Source: CAD feature listing. Evaluate the final solid. Frame: model axes, mm. Coordinates: 2 decimals unless noted, no trailing zeros. Loops run counter-clockwise (first coordinate to the right, second up) from the corner with the lowest first, then second, coordinate; pieces in that order, holes last. Notation, with made-up numbers: (-30, 16) -> (18, 16) arc R15 ccw to (18, 40) -> close; hole circle Ø1 at (85.25, 2.5). An arc over 180 degrees is marked (long way). Answer as CSV lines item,"result".
from build123d import *

# Parameters (mm, degrees)
SKETCH1_R                                    = 32
SKETCH1_R_2                                  = 8.25
BOSS_EXTRUDE1_DEPTH                          = 2
CSK_FOR_M3_HEX_SOCKET_COUNTERSUNK_HE_2_COUNT = 2
CSK_FOR_M3_HEX_SOCKET_COUNTERSUNK_HE_2_PITCH = 15
CSK_FOR_M3_HEX_SOCKET_COUNTERSUNK_HE_3_COUNT = 2
CSK_FOR_M3_HEX_SOCKET_COUNTERSUNK_HE_3_PITCH = 25.980762114
CSK_FOR_M3_HEX_SOCKET_COUNTERSUNK_HE_4_COUNT = 2
CSK_FOR_M3_HEX_SOCKET_COUNTERSUNK_HE_4_PITCH = 30
CSK_FOR_M3_HEX_SOCKET_COUNTERSUNK_HE_5_COUNT = 2
CSK_FOR_M3_HEX_SOCKET_COUNTERSUNK_HE_5_PITCH = 25.980762114
CSK_FOR_M3_HEX_SOCKET_COUNTERSUNK_HE_6_COUNT = 2
CSK_FOR_M3_HEX_SOCKET_COUNTERSUNK_HE_6_PITCH = 15
M3_CLEARANCE_HOLE1_D                         = 3.6


with BuildPart() as part:
    # Sketch1 → Boss-Extrude1 (new body)
    with BuildSketch(Plane(origin=(0, 0, 0), x_dir=(1, 0, 0), z_dir=(0, 1, 0))):
        with Locations(Location((0, 0, 0), (0, 0, 270))):
            Circle(SKETCH1_R)
        with Locations(Location((0, 0, 0), (0, 0, 270))):
            Circle(SKETCH1_R_2, mode=Mode.SUBTRACT)
    extrude(amount=BOSS_EXTRUDE1_DEPTH)

    # Sketch4 → CSK for M3 Hex Socket Countersunk Head Screw1 (revolve, cut)
    with BuildSketch(Plane(origin=(-7.5, 0, -12.990381057), x_dir=(0, 0, -1), z_dir=(1, 0, 0))):
        Polygon((0, 0), (0, 2), (1.7, 2), (1.7, 1.05), (2.75, 0), align=None)
    csk_for_m3_hex_socket_countersunk_head_s = revolve(axis=Axis((-7.5, -6.35, -12.990381057), (0, 1, 0)), mode=Mode.SUBTRACT)

    # CSK for M3 Hex Socket Countersunk He 2: CSK for M3 Hex Socket Countersunk Head Screw1 ×2
    with Locations(*[(i * CSK_FOR_M3_HEX_SOCKET_COUNTERSUNK_HE_2_PITCH, 0, 0) for i in range(1, CSK_FOR_M3_HEX_SOCKET_COUNTERSUNK_HE_2_COUNT)]):
        add(csk_for_m3_hex_socket_countersunk_head_s, mode=Mode.SUBTRACT)

    # CSK for M3 Hex Socket Countersunk He 3: CSK for M3 Hex Socket Countersunk Head Screw1 ×2
    with Locations(*[Vector(0.8660254037844752, 0, 0.49999999999993666) * (i * CSK_FOR_M3_HEX_SOCKET_COUNTERSUNK_HE_3_PITCH) for i in range(1, CSK_FOR_M3_HEX_SOCKET_COUNTERSUNK_HE_3_COUNT)]):
        add(csk_for_m3_hex_socket_countersunk_head_s, mode=Mode.SUBTRACT)

    # CSK for M3 Hex Socket Countersunk He 4: CSK for M3 Hex Socket Countersunk Head Screw1 ×2
    with Locations(*[Vector(0.5000000000000633, 0, 0.8660254037844022) * (i * CSK_FOR_M3_HEX_SOCKET_COUNTERSUNK_HE_4_PITCH) for i in range(1, CSK_FOR_M3_HEX_SOCKET_COUNTERSUNK_HE_4_COUNT)]):
        add(csk_for_m3_hex_socket_countersunk_head_s, mode=Mode.SUBTRACT)

    # CSK for M3 Hex Socket Countersunk He 5: CSK for M3 Hex Socket Countersunk Head Screw1 ×2
    with Locations(*[(0, 0, i * CSK_FOR_M3_HEX_SOCKET_COUNTERSUNK_HE_5_PITCH) for i in range(1, CSK_FOR_M3_HEX_SOCKET_COUNTERSUNK_HE_5_COUNT)]):
        add(csk_for_m3_hex_socket_countersunk_head_s, mode=Mode.SUBTRACT)

    # CSK for M3 Hex Socket Countersunk He 6: CSK for M3 Hex Socket Countersunk Head Screw1 ×2
    with Locations(*[Vector(-0.499999999999937, 0, 0.8660254037844751) * (i * CSK_FOR_M3_HEX_SOCKET_COUNTERSUNK_HE_6_PITCH) for i in range(1, CSK_FOR_M3_HEX_SOCKET_COUNTERSUNK_HE_6_COUNT)]):
        add(csk_for_m3_hex_socket_countersunk_head_s, mode=Mode.SUBTRACT)

    # M3 Clearance Hole1 (through all)
    with Locations(Plane(origin=(0, 0, 0), x_dir=(-1, 0, 0), z_dir=(0, -1, 0))):
        with Locations((-12, -20.784609691), (-24, 0), (-12, 20.784609691), (12, 20.784609691), (24, 0), (12, -20.784609691)):
            Hole(M3_CLEARANCE_HOLE1_D / 2)


solid = part.part
(1) Material intervals for L1, parallel to X at y = 1.2, z = -13.5; L2, parallel to Z at x = -12, y = 0.75; L3, parallel to Z at x = -7.5, y = 1.5, sorted ascending. Write a range as [from, to].
Computed values:
L1,"[-29.01, -9.12], [-5.88, 5.88], [9.12, 29.01]"
L2,"[-29.66, -22.58], [-18.98, 18.98], [22.58, 29.66]"
L3,"[-31.11, -14.69], [-11.29, -3.44], [3.44, 11.29], [14.69, 31.11]"
(2) Cut plane C-C (y = 1.55). State how many separate pieces and enclosed holes the cut face has, then the cut area to 3 significant figures.
Computed values:
separate pieces,"1"
enclosed holes,"13"
area,"2,890 mm^2"
(3) Draft query along Z for faces 1 (the cylindrical face through (-22.283, 1.014, -0.541)), 2 (the flat face through (-7, 2, 7)), 3 (the cylindrical face through (-31.24, 0.99, -6.94)). Return one class per face: released by +Z, released by -Z, zero draft, split by the parting line, or undercut.
Computed values:
face 1,"undercut"
face 2,"zero draft"
face 3,"split by the parting line"
(4) Cut plane B-B (z = 4). Return the cut outline in (x, y).
Computed values:
outline,"(-31.75, 0) -> (-7.22, 0) -> (-7.22, 2) -> (-31.75, 2) -> close; (7.22, 0) -> (31.75, 0) -> (31.75, 2) -> (7.22, 2) -> close"
(5) Cut plane A-A (x = 0). Return the cut outline in (y, z).
Computed values:
outline,"(0, -32) -> (2, -32) -> (2, -8.25) -> (0, -8.25) -> close; (0, 8.25) -> (2, 8.25) -> (2, 32) -> (0, 32) -> close"
(6) Cut plane D-D (x = -7.5). Return the cut outline in (y, z).
Computed values:
outline,"(0, -31.11) -> (2, -31.11) -> (2, -14.69) -> (1.05, -14.69) -> (0, -15.74) -> close; (0, -10.24) -> (1.05, -11.29) -> (2, -11.29) -> (2, -3.44) -> (0, -3.44) -> close; (0, 3.44) -> (2, 3.44) -> (2, 11.29) -> (1.05, 11.29) -> (0, 10.24) -> close; (0, 15.74) -> (1.05, 14.69) -> (2, 14.69) -> (2, 31.11) -> (0, 31.11) -> close"
(7) Pin query (flat end, axial travel): pin 1 Ø2 at (x, z) = (-25, -23.5) entering from +Y; pin 2 Ø4.5 at (x, z) = (-15, 0) entering from -Y. Return the tip coordinate at first contact, or that it passes through.
Computed values:
pin 1,"through"
pin 2,"y = 0.5"
